Input: dimensioned drawing with shaded views. Units: mm. Origin: part minimum x, y, z. A direction names the side the tool comes from. Round coordinates to 2 decimals unless told otherwise and drop trailing zeros. Write each loop counter-clockwise with the first axis right and the second up, starting at its lowest first coordinate (ties: lowest second). Pieces come first, ordered by that corner, then holes. Notation, with made-up numbers: (16, -5) -> (61, -5) arc R30 cw to (61, 34) -> close; hole circle Ø3 at (56.5, 81.25). An arc over 180 degrees is marked (long way). Use one line per item in the form item = value. Start each with the question number.
1. Draft query along Y for the marked faces 1, 2 and 3. Return one class per face: pulls with the +Y half, pulls with the -Y half, needs draft (parallel to the pull), parting line crosses it, or undercut.
2. Cut plane C-C, the plane x = 45. Return the cut outline in (y, z) (1 decimal).
3. Pin query (flat end, axial travel): pin 1 Ø8 at (x, z) = (50.5, 14) entering from +Y; pin 2 Ø3.5 at (x, z) = (55, 10.5) entering from -Y (1 decimal); pin 3 Ø12 at (y, z) = (33.5, 6) entering from -X; pin 4 Ø4 at (y, z) = (9.5, 2.5) entering from -X (1 decimal). Return the tip coordinate at first contact, or that it passes through.
4. Cut plane B-B, the plane z = 9.5. Return the cut outline in (x, y) (1 decimal), plus the area to 3 significant figures.
5. Cut plane A-A, the plane y = 53.5. Return the cut outline in (x, z).
6. Reachability of the marked faces 4, 5 and 6 from +Z, -Z, +X, -X, +Y, -Y: full face, straight path, thin tool, end or side. Return the list, or none.
7. Line query: L1, parallel to X at y = 30.5, z = 2.25; L2, parallel to X at y = 10, z = 8.25; L3, parallel to Y at x = 15, z = 15.5. Output: solid intervals per line, ascending.
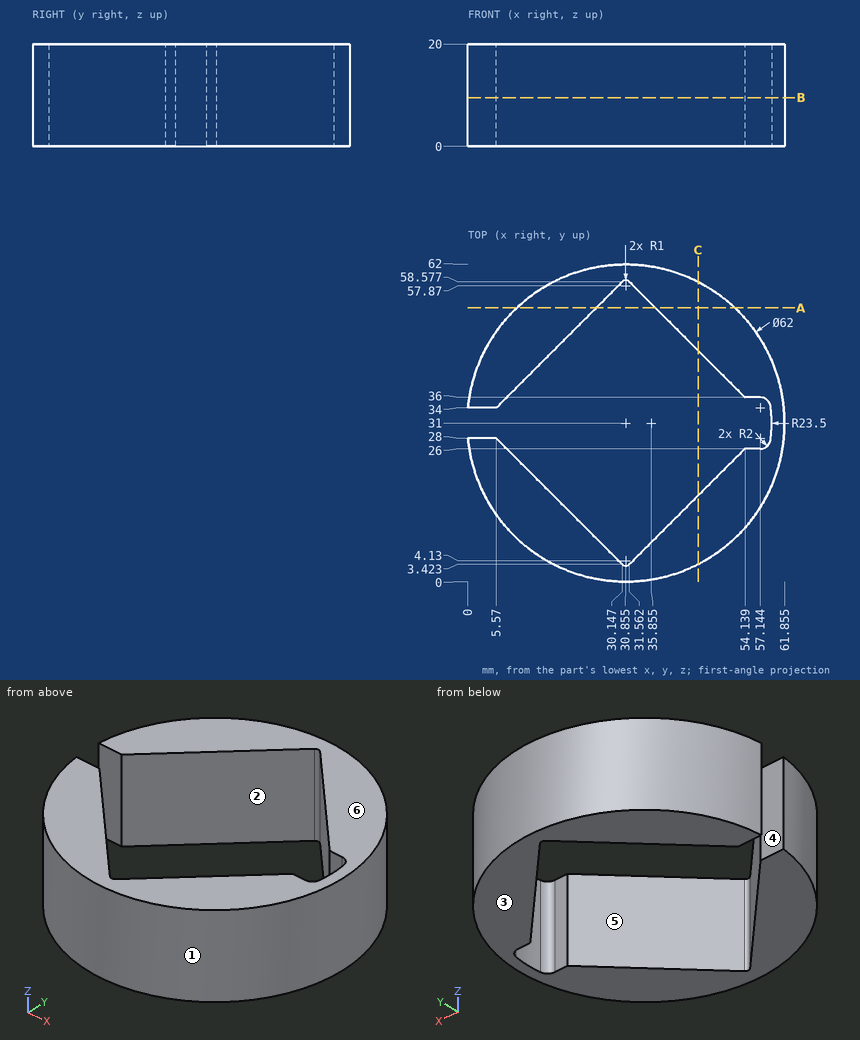
Outcome:
q1.face_1 = parting line crosses it
q1.face_2 = undercut
q1.face_3 = needs draft
q2.outline = (3.4, 0) -> (16.9, 0) -> (16.9, 20) -> (3.4, 20) -> close; (45.1, 0) -> (58.6, 0) -> (58.6, 20) -> (45.1, 20) -> close
q3.pin_1 = 57.76
q3.pin_2 = 9.6
q3.pin_3 = 0
q3.pin_4 = 6.8
q4.outline = (0, 28) arc R31 ccw (long way) to (0, 34) -> (5.6, 34) -> (30.1, 58.6) arc R1 cw to (31.6, 58.6) -> (54.1, 36) -> (57.1, 36) arc R2 cw to (59.1, 34.3) arc R23.5 cw to (59.1, 27.7) arc R2 cw to (57.1, 26) -> (54.1, 26) -> (31.6, 3.4) arc R1 cw to (30.1, 3.4) -> (5.6, 28) -> close
q4.area = 1,370 mm^2
q5.outline = (9.53, 0) -> (25.07, 0) -> (25.07, 20) -> (9.53, 20) -> close; (36.64, 0) -> (52.18, 0) -> (52.18, 20) -> (36.64, 20) -> close
q6.face_4 = +Z, -Z, -X
q6.face_5 = +Z, -Z
q6.face_6 = +Z, +X, -X, +Y, -Y
q7.L1 = 59.35 to 61.85
q7.L2 = 8.05 to 23.57, 38.14 to 53.66
q7.L3 = 4.36 to 18.57, 43.43 to 57.64
